CAD build for the part. Positions are in the model's coordinates, mm. A direction names the side the tool comes from. Give positions to 0.01 mm unless a question says otherwise; leave off trailing zeros. Write each loop counter-clockwise with the first axis right and the second up, starting at its lowest first coordinate (ties: lowest second). Pieces come first, ordered by that corner, then holes. Notation, with made-up numbers: M 16.25,46.25 L 56.25,46.25 A30 ccw 56.25,76.25 Z; hole C 43.5,55.5 d1. An arc over 180 degrees is marked long. One line per question, with ' | ' between items. Start each with the question number.
1. Which spindle directions (+Z, -Z, +X, -X, +Y, -Y) get a long thin tool onto all of the face, cutting with end or side? Do faces 1 (the face through (-212, -38, 64.137)), 2 (the face through (-205.695, -38, 70)), 3 (the face through (-75, -38, 12.7)). Say none if no direction does.
2. Cut at D-D, the plane y = -70. Write the cut outline in (x, z), then the cut area to 3 significant figures.
3. Pull direction X, two halves, no side cores. Call faces 4 (the face through (0, -38, 28)), 5 (the face through (-52, -38, 57.628)), 6 (the face through (-173, -38, 64.137)): released by +X, released by -X, zero draft, split by the parting line, or undercut.
4. Flat gauge pins, fed straight in: pin 1 (6.5 mm diameter, centred on y = -30.5, z = 4.5, fed in from +X); pin 2 (4 mm diameter, centred on y = -34, z = 69, fed in from +X); pin 3 (5 mm diameter, centred on y = -60, z = 20, fed in from +X); pin 4 (1 mm diameter, centred on x = -65.5, y = -32, fed in from +Z). Where does each tip first touch, or does it go through?
5. Cut at B-B, the plane y = -28. Write the cut outline in (x, z), then the cut area to 3 significant figures.
6. Wall check: L1, parallel to Z at x = -211, y = -24; L2, parallel to X at y = -66, z = 55; L3, parallel to X at y = -25, z = 6.5. Give the ranges that are in metal, low to high.
7. Cut at C-C, the plane x = -85.5. Write the cut outline in (y, z).
8. Cut at A-A, the plane z = 55.5. Write the cut outline in (x, y).
```python
from build123d import *

# Parameters (mm, degrees)
F1_DEPTH = 76.2
F3_DEPTH = 152.4


with BuildPart() as f1:
    # F0 (on Front) → F1 (new body)
    with BuildSketch(Plane.XZ):
        Polygon((-230.51038, 0), (0, 0), (0, 57.627595), (-105.650591, 57.627595), (-115.25519, 76.836793), (-178.560193, 76.836793), (-178.560193, 64.136793), (-167.302838, 64.136793), (-167.302838, 51.436793), (-218.102838, 51.436793), (-218.102838, 64.136793), (-205.695296, 64.136793), (-205.695296, 76.836793), (-230.51038, 76.836793), align=None)
    extrude(amount=F1_DEPTH)

    # F2 (on face) → F3 (cut)
    with BuildSketch(Plane.YZ):
        Polygon((-12.7, 12.7), (-38.1, 12.7), (-63.5, 12.7), (-50.8, 0), (-25.4, 0), align=None)
    extrude(amount=-F3_DEPTH, mode=Mode.SUBTRACT)


solid = f1.part
```
Here are the results:
1) face 1: +Y, -Y | face 2: +Z, +Y, -Y | face 3: +X
2) outline: M -230.51,0 L 0,0 L 0,57.63 L -105.65,57.63 L -115.26,76.84 L -178.56,76.84 L -178.56,64.14 L -167.3,64.14 L -167.3,51.44 L -218.1,51.44 L -218.1,64.14 L -205.7,64.14 L -205.7,76.84 L -230.51,76.84 Z | area: 14,600 mm^2
3) face 4: released by +X | face 5: zero draft | face 6: undercut
4) pin 1: x = -152.4 | pin 2: x = -110.34 | pin 3: x = 0 | pin 4: z = 57.63
5) outline: M -230.51,0 L -152.4,0 L -152.4,12.7 L 0,12.7 L 0,57.63 L -105.65,57.63 L -115.26,76.84 L -178.56,76.84 L -178.56,64.14 L -167.3,64.14 L -167.3,51.44 L -218.1,51.44 L -218.1,64.14 L -205.7,64.14 L -205.7,76.84 L -230.51,76.84 Z | area: 12,700 mm^2
6) L1: 0 to 51.44, 64.14 to 76.84 | L2: -230.51 to -218.1, -167.3 to 0 | L3: -230.51 to -152.4
7) outline: M -76.2,0 L -50.8,0 L -63.5,12.7 L -12.7,12.7 L -25.4,0 L 0,0 L 0,57.63 L -76.2,57.63 Z
8) outline: M -230.51,-76.2 L -218.1,-76.2 L -218.1,0 L -230.51,0 Z; M -167.3,-76.2 L 0,-76.2 L 0,0 L -167.3,0 Z
